The figure shows three views and two pictorial views of one solid part (mm, origin at its lowest corner). Answer the questions. A direction names the side the tool comes from. Coordinates: 2 decimals unless noted, no trailing zeros. Write each loop counter-clockwise with the first axis right and the second up, starting at its lowest first coordinate (ties: lowest second). Pieces come first, ordered by that corner, then holes.
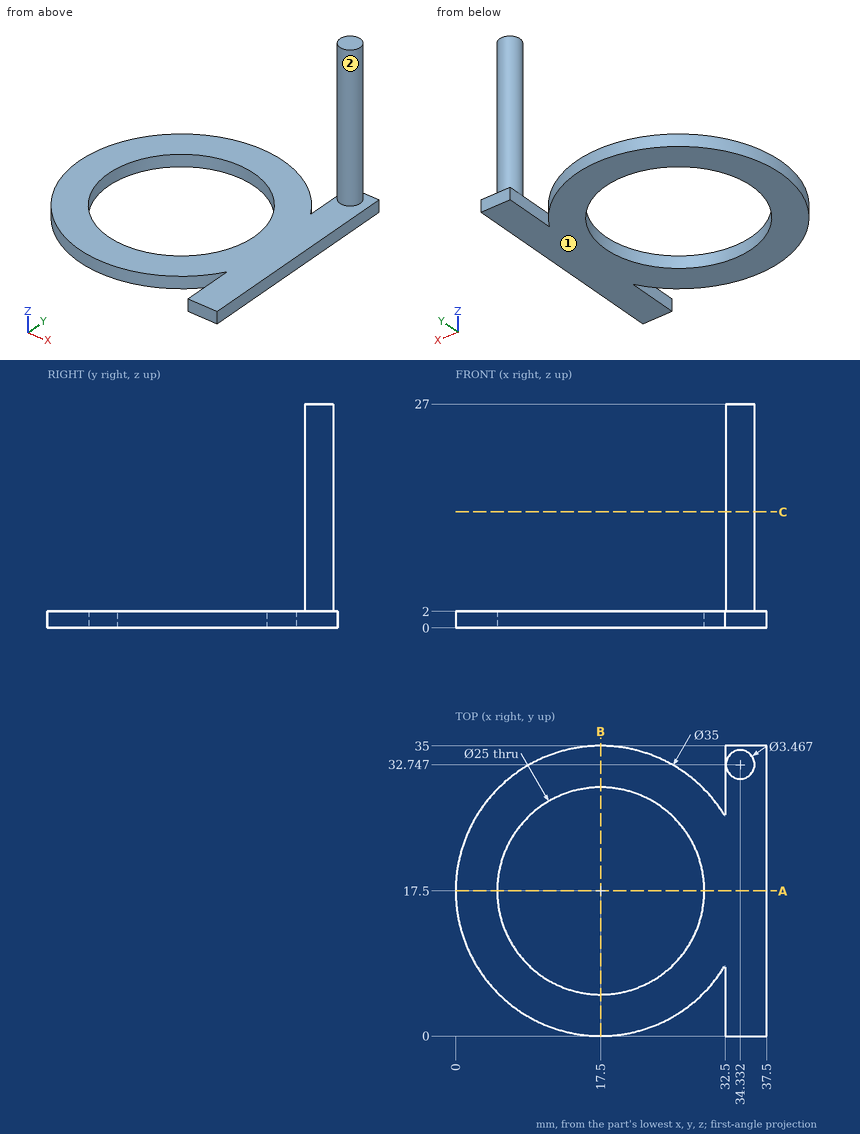
1. Section C-C on z = 14 is taken. Give the vertices of the cut face in (x, y) (1 decimal).
Results found:
outline: circle Ø3.5 at (34.3, 32.7)
2. Section B-B on x = 17.5 is taken. Give the vertices of the cut face in (y, z).
Results found:
outline: (0, 0) - (5, 0) - (5, 2) - (0, 2) - close; (30, 0) - (35, 0) - (35, 2) - (30, 2) - close
3. A tool of negligible diameter and unlimited length cuts with its end or side. For the marked faces 1 and 2, from which of +Z, -Z, +X, -X, +Y, -Y can it reach the whole face along a straight path? Write none if from no direction.
Results found:
face 1: -Z, +X, -X, +Y, -Y
face 2: +Z
4. Find the intervals of material crossed by L1, parallel to Y at x = 17.5, z = 0.45; L2, parallel to Z at x = 31.5, y = 18; L3, parallel to X at y = 33, z = 14, in increasing order.
Results found:
L1: y = 0 to 5, 30 to 35
L2: z = 0 to 2
L3: x = 32.62 to 36.05
5. Section A-A on y = 17.5 is taken. Give the vertices of the cut face in (x, z), then the cut area to 3 significant figures.
Results found:
outline: (0, 0) - (5, 0) - (5, 2) - (0, 2) - close; (30, 0) - (37.5, 0) - (37.5, 2) - (30, 2) - close
area: 25.0 mm2
6. Flat-ended cylindrical pins translate along their axes: P1, Ø4, axis at y = 28.5, z = 16.5, coming from the +X side; P2, Ø2, axis at y = 31, z = 0.5, coming from the -X side; P3, Ø1.6, axis at y = 3.5, z = 0.5, coming from the -X side; P4, Ø1, axis at x = 29.5, y = 24.5, coming from the +Z side. Find the tip coordinate at first contact, or state that the pin passes through.
Results found:
P1: passes through
P2: stops at x = 5.25
P3: stops at x = 6.01
P4: stops at z = 2
